from build123d import *

# Parameters (mm, degrees)
SKETCH1_R           = 35.56
BOSS_EXTRUDE1_DEPTH = 1.5875
SKETCH2_W           = 1.5875
SKETCH2_H           = 6.35
CUT_EXTRUDE1_DEPTH  = 51.389560675
CIRPATTERN1_COUNT   = 8
BOSS_EXTRUDE2_DEPTH = 3.175
SKETCH4_R           = 1.397
CUT_EXTRUDE2_DEPTH  = 3.175
CIRPATTERN2_COUNT   = 4
CUT_EXTRUDE3_DEPTH  = 51.339522371
CIRPATTERN3_COUNT   = 8
SKETCH6_R           = 1.397
CUT_EXTRUDE4_DEPTH  = 51.339522371
CIRPATTERN4_COUNT   = 16


with BuildPart() as part:
    # Sketch1 → Boss-Extrude1 (new, symmetric)
    with BuildSketch(Plane(origin=(0, 0, 0), x_dir=(1, 0, 0), z_dir=(0, 1, 0))):
        with Locations(Location((0, 0, 0), (0, 0, 270))):
            Circle(SKETCH1_R)
        with BuildLine():
            ThreePointArc((-13.969422727, 0.126998688), (-11.005254984, 8.604955708), (-3.4925, 13.526394337))
            Line((-3.4925, 13.526394337), (-3.4925, 14.351))
            Line((-3.4925, 14.351), (3.4925, 14.351))
            Line((3.4925, 14.351), (3.4925, 13.526394337))
            ThreePointArc((3.4925, 13.526394337), (11.044254728, 8.554842927), (13.97, 0))
            ThreePointArc((13.97, 0), (0.0635, -13.969855681), (-13.969422727, -0.126998688))
            ThreePointArc((-13.969422727, -0.126998688), (-14.097, 0), (-13.969422727, 0.126998688))
        make_face(mode=Mode.SUBTRACT)
    extrude(amount=BOSS_EXTRUDE1_DEPTH, both=True)

    # Sketch2 → Cut-Extrude1 (cut, through all)
    with BuildSketch(Plane(origin=(0, 1.5875, 0), x_dir=(1, 0, 0), z_dir=(0, 1, 0))):
        with BuildLine():
            ThreePointArc((1.5875, 35.524547059), (0.793947914, 35.55113566), (0, 35.56))
            Line((0, 35.56), (0, 29.174547059))
            Line((0, 29.174547059), (1.5875, 29.174547059))
            Line((1.5875, 29.174547059), (1.5875, 35.524547059))
        make_face()
        with BuildLine():
            Line((0, 29.174547059), (0, 35.56))
            ThreePointArc((0, 35.56), (-0.793947914, 35.55113566), (-1.5875, 35.524547059))
            Line((-1.5875, 35.524547059), (-1.5875, 29.174547059))
            Line((-1.5875, 29.174547059), (0, 29.174547059))
        make_face()
        with Locations((-0.79375, 19.649547059)):
            Rectangle(SKETCH2_W, SKETCH2_H)
        with Locations((0.79375, 19.649547059)):
            Rectangle(SKETCH2_W, SKETCH2_H)
    cut_extrude1 = extrude(amount=-CUT_EXTRUDE1_DEPTH, mode=Mode.SUBTRACT)

    # CirPattern1: Cut-Extrude1 ×8 about axis
    cirpattern1_axis = Axis((0, 0, 0), (0, 1, 0))
    for i in range(1, CIRPATTERN1_COUNT):
        add(cut_extrude1.rotate(cirpattern1_axis, i * 360 / CIRPATTERN1_COUNT), mode=Mode.SUBTRACT)

    # Sketch3 → Boss-Extrude2 (add)
    with BuildSketch(Plane(origin=(0, 1.5875, 0), x_dir=(1, 0, 0), z_dir=(0, 1, 0))):
        with BuildLine():
            ThreePointArc((-13.969422727, -0.126998688), (-13.905725148, -1.338547016), (-13.73715036, -2.54))
            Line((-13.73715036, -2.54), (-10.81615036, -2.54))
            Line((-10.81615036, -2.54), (-10.81615036, 8.84148129))
            ThreePointArc((-10.81615036, 8.84148129), (-13.1364649, 4.753334612), (-13.969422727, 0.126998688))
            ThreePointArc((-13.969422727, 0.126998688), (-14.097, 0), (-13.969422727, -0.126998688))
        make_face()
        with BuildLine():
            Line((10.68915036, -2.54), (13.73715036, -2.54))
            ThreePointArc((13.73715036, -2.54), (13.506399758, 3.569042671), (10.68915036, 8.994607528))
            Line((10.68915036, 8.994607528), (10.68915036, -2.54))
        make_face()
        with BuildLine():
            Line((2.794, -8.89), (2.794, -13.687748683))
            ThreePointArc((2.794, -13.687748683), (7.196729012, -11.973637356), (10.776307345, -8.89))
            Line((10.776307345, -8.89), (2.794, -8.89))
        make_face()
        with BuildLine():
            Line((-2.794, -8.89), (-10.776307345, -8.89))
            ThreePointArc((-10.776307345, -8.89), (-7.196729012, -11.973637356), (-2.794, -13.687748683))
            Line((-2.794, -13.687748683), (-2.794, -8.89))
        make_face()
    extrude(amount=-BOSS_EXTRUDE2_DEPTH)

    # Sketch4 → Cut-Extrude2 (cut)
    with BuildSketch(Plane(origin=(0, 1.5875, 0), x_dir=(1, 0, 0), z_dir=(0, 1, 0))):
        with Locations(Location((7.544056765, 18.212964157, 0), (0, 0, 270))):
            Circle(SKETCH4_R)
    cut_extrude2 = extrude(amount=-CUT_EXTRUDE2_DEPTH, mode=Mode.SUBTRACT)

    # CirPattern2: Cut-Extrude2 ×4 about axis
    cirpattern2_axis = Axis((0, 0, 0), (0, 1, 0))
    for i in range(1, CIRPATTERN2_COUNT):
        add(cut_extrude2.rotate(cirpattern2_axis, i * 360 / CIRPATTERN2_COUNT), mode=Mode.SUBTRACT)

    # Sketch5 → Cut-Extrude3 (cut, through all)
    with BuildSketch(Plane(origin=(0, 1.5875, 0), x_dir=(1, 0, 0), z_dir=(0, 1, 0))):
        Polygon((-26.379011196, 12.644841817), (-27.594031094, 9.711524302), (-21.727396062, 7.281484506), (-20.512376164, 10.214802022), align=None)
    cut_extrude3 = extrude(amount=-CUT_EXTRUDE3_DEPTH, mode=Mode.SUBTRACT)

    # CirPattern3: Cut-Extrude3 ×8 about axis
    cirpattern3_axis = Axis((0, 0, 0), (0, 1, 0))
    for i in range(1, CIRPATTERN3_COUNT):
        add(cut_extrude3.rotate(cirpattern3_axis, i * 360 / CIRPATTERN3_COUNT), mode=Mode.SUBTRACT)

    # Sketch6 → Cut-Extrude4 (cut, through all)
    with BuildSketch(Plane(origin=(0, 1.5875, 0), x_dir=(1, 0, 0), z_dir=(0, 1, 0))):
        with Locations(Location((-16.075914933, 24.065531637, 0), (0, 0, 270))):
            Circle(SKETCH6_R)
    cut_extrude4 = extrude(amount=-CUT_EXTRUDE4_DEPTH, mode=Mode.SUBTRACT)

    # CirPattern4: Cut-Extrude4 ×16 about axis
    cirpattern4_axis = Axis((0, 0, 0), (0, 1, 0))
    for i in range(1, CIRPATTERN4_COUNT):
        add(cut_extrude4.rotate(cirpattern4_axis, i * 360 / CIRPATTERN4_COUNT), mode=Mode.SUBTRACT)


solid = part.part
The listing builds one solid part. Answer for the finished solid, in the listing's coordinates (mm). A direction names the side the tool comes from. Coordinates: 2 decimals unless noted, no trailing zeros. Use one line per item in the form item = value.
Item 1: For faces 1 (the face through (0, 0, -22.825)), 2 (the face through (0, 0, -29.175)), 3 (the face through (13.45, 0.02, 32.92)), 4 (the face through (29.175, 0, 0)), determine the directions among +Z, -Z, +X, -X, +Y, -Y from which every point of the face is accessible in a straight line to the end or side of a thin tool.
Model answer:
face_1 = +Y, -Y
face_2 = -Z, +Y, -Y
face_3 = +Z, +X, +Y, -Y
face_4 = +X, +Y, -Y
Item 2: Find section B-B, the plane y = -0.55. Give the number of separate pieces and of enclosed holes in the cut face, plus the area to 3 significant figures.
Model answer:
separate_pieces = 1
enclosed_holes = 37
area = 2,850 mm2
Item 3: Find the intervals of material crossed by probe 1 along Z at (x, y) = (-24.5, 0.8); probe 2 along Z at (x, y) = (4.5, 1); probe 3 along X at (y, z) = (-0.45, -20), in increasing order.
Model answer:
probe_1 = -22.25 to -17.41, -14.76 to -11.87, -8.43 to 8.43, 11.87 to 14.75, 17.4 to 22.25
probe_2 = -35.27 to -29.18, -27.59 to -13.23, 8.89 to 27.58, 29.19 to 35.27
probe_3 = -29.4 to -22.25, -21.26 to -1.59, 1.59 to 21.26, 22.25 to 29.4
Item 4: Given P1, Ø2.5, axis at x = 16.08, z = 24.07, coming from the +Y side; P2, Ø1, axis at y = -1, z = -19, coming from the -X side; P3, Ø1.6, axis at x = -7, y = 0, coming from the -Z side; P4, Ø1, axis at y = 0, z = -31.5, coming from the +X side, each flat-ended and moving along its own axis, determine where each tip first touches the part or whether it passes through.
Model answer:
P1 = through
P2 = -30.37
P3 = -35.02
P4 = 17.42
